from build123d import *

# Parameters (mm, degrees)
SKETCH2_W          = 118.314728146
SKETCH2_H          = 12
CUT_EXTRUDE1_DEPTH = 10
SKETCH3_W          = 4
SKETCH3_H          = 6
CUT_EXTRUDE2_DEPTH = 80.962050875
FILLET1_R          = 5


with BuildPart() as part:
    # Sketch1 → Revolve1 (revolve)
    with BuildSketch(Plane(origin=(0, 0, 0), x_dir=(0, 0, -1), z_dir=(1, 0, 0)), mode=Mode.PRIVATE) as revolve1_sk:
        Polygon((0, 15), (0, 44.124423963), (-20, 44.124423963), (-20, 29.746543779), (-50, 29.746543779), (-50, 15), align=None)
    revolve(revolve1_sk.sketch.rotate(Axis((0, 0, 0), (0, 0, 1)), 90), axis=Axis((0, 0, 0), (0, 0, 1)))

    # Sketch2 → Cut-Extrude1 (cut)
    with BuildSketch(Plane(origin=(0, 0, 0), x_dir=(-1, 0, 0), z_dir=(0, 0, -1))):
        Rectangle(SKETCH2_W, SKETCH2_H)
    extrude(amount=-CUT_EXTRUDE1_DEPTH, mode=Mode.SUBTRACT)

    # Sketch3 → Cut-Extrude2 (cut, through all)
    with BuildSketch(Plane.XY.offset(50)):
        with Locations((16, 0)):
            Rectangle(SKETCH3_W, SKETCH3_H)
    extrude(amount=-CUT_EXTRUDE2_DEPTH, mode=Mode.SUBTRACT)

    # Fillet1
    fillet1_edges = [part.edges().sort_by_distance(p)[0] for p in [
        (29.746543779, 0, 20),
    ]]
    fillet(fillet1_edges, radius=FILLET1_R)


solid = part.part
Geometry check sheet. Reference: the model listing, model coordinates, mm. A direction names the side the tool comes from. Round coordinates to 2 decimals unless told otherwise and drop trailing zeros. Order: outer loops, then holes, each group sorted by start corner. A loop starts at its lowest first (then second) coordinate and runs counter-clockwise, first axis right, second up. Notation, with made-up numbers: (-38, -11.5) -> (-34, -11.5) arc R33 cw to (-34, 18.5) -> close; hole circle Ø9 at (6.25, -8). An arc over 180 degrees is marked (long way). Use one line per item in the form item = value.
1. Cross-section at B-B, the plane y = 0. Enter the section's corners in (x, z).
Working result:
outline = (-44.12, 10) -> (-15, 10) -> (-15, 50) -> (-29.75, 50) -> (-29.75, 25) arc R5 cw to (-34.75, 20) -> (-44.12, 20) -> close; (18, 10) -> (44.12, 10) -> (44.12, 20) -> (34.75, 20) arc R5 cw to (29.75, 25) -> (29.75, 50) -> (18, 50) -> close
2. Go/stop test with flat-tipped pins: pin 1 (6 mm diameter, centred on x = -2.5, y = -9.5, fed in from +Z); pin 2 (3 mm diameter, centred on y = 0, z = 31, fed in from -X); pin 3 (1 mm diameter, centred on y = 18.5, z = 35.5, fed in from -X); pin 4 (2 mm diameter, centred on x = 1.5, z = 17.5, fed in from -Y). Record where each tip stops, or that it passes through.
Working result:
pin_1 = through
pin_2 = -29.75
pin_3 = -23.68
pin_4 = -44.12
3. Mould release check, pull along Y, two halves, no side actions. Record for faces 1 (the face through (-29, -6, 5)), 2 (the face through (-12.9, 32.5, 20)), 3 (the face through (-40.76, 16.9, 10.14)): pulls with the +Y half, pulls with the -Y half, needs draft (parallel to the pull), parting line crosses it, or undercut.
Working result:
face_1 = undercut
face_2 = needs draft
face_3 = parting line crosses it
4. Set-up check for faces 4 (the face through (16, 3, 30)), 5 (the face through (-28.37, -8.94, 37.67)), 6 (the face through (-1, 25, 0)), 7 (the face through (-29, 0, 10)): record each of +Z, -Z, +X, -X, +Y, -Y from which the full face is reachable in a straight line by a thin tool's end or side.
Working result:
face_4 = +Z, -Z
face_5 = +Z
face_6 = -Z, +X, -X, +Y, -Y
face_7 = -Z, +X, -X
5. Cross-section at D-D, the plane x = 37.5. Enter the section's corners in (y, z), plus the area to 3 significant figures.
Working result:
outline = (-23.25, 0) -> (-6, 0) -> (-6, 10) -> (6, 10) -> (6, 0) -> (23.25, 0) -> (23.25, 20) -> (-23.25, 20) -> close
area = 810 mm^2
6. Scan lines: line 1 along Y through (x, z) = (0, 17.5); line 2 along Y through (x, z) = (0, 37.5); line 3 along Z through (x, y) = (-29.5, -20.5). Record each from-to range of solid material in increasing order. Write a range as from..to.
Working result:
line_1 = -44.12..-15, 15..44.12
line_2 = -29.75..-15, 15..29.75
line_3 = 0..20
7. Cross-section at C-C, the plane z = 40. Enter the section's corners in (x, y), plus the area to 3 significant figures.
Working result:
outline = circle Ø59.49 at (0, 0); hole (14.7, -3) -> (18, -3) -> (18, 3) -> (14.7, 3) arc R15 ccw (long way) to start
area = 2,050 mm^2
8. Cross-section at A-A, the plane x = 0. Enter the section's corners in (y, z), plus the area to 3 significant figures.
Working result:
outline = (-44.12, 0) -> (-15, 0) -> (-15, 50) -> (-29.75, 50) -> (-29.75, 25) arc R5 cw to (-34.75, 20) -> (-44.12, 20) -> close; (15, 0) -> (44.12, 0) -> (44.12, 20) -> (34.75, 20) arc R5 cw to (29.75, 25) -> (29.75, 50) -> (15, 50) -> close
area = 2,060 mm^2
